Here's the drawing with two shaded views (mm, measured from the low corner). I have some questions. A direction names the side the tool comes from. Round coordinates to 2 decimals unless told otherwise and drop trailing zeros. Loops run counter-clockwise (first coordinate to the right, second up) from the corner with the lowest first, then second, coordinate; pieces in that order, holes last.
(1) Thinking about a two-plate mould opening in Z: for the marked faces 3, 4, 5 and 6, which applies, released by +Z, released by -Z, zero draft, split by the parting line, or undercut?
(2) I want a section at A-A on z = 12.7. Write out the boundary of the cut face in (x, y) (3 decimals).
(3) I want a section at B-B on y = 38. Write out the boundary of the cut face in (x, z) (3 decimals).
(4) If I drill on line 1 along Y through (x, z) = (24.25, 12); line 2 along X through (y, z) = (46.5, 7) (3 decimals); line 3 along Y through (x, z) = (26.5, 11), over which ranges is the centre line in solid material (lowest first)?
(5) I want a section at C-C on x = 12. Write out the boundary of the cut face in (y, z).
(6) Will these pins go through, and if not, where does the flat tip stop? pin 1 Ø7.5 at (y, z) = (48.5, 11.5) entering from -X; pin 2 Ø4 at (x, z) = (24, 12) entering from -Y; pin 3 Ø7.5 at (x, z) = (6.5, 12.5) entering from +Y.
(7) I want a section at D-D on z = 23.25. Write out the boundary of the cut face in (x, y) (3 decimals).
(8) Which directions (+Z, -Z, +X, -X, +Y, -Y) give clear straight access to the entire face, cutting with the end or side of a thin tool? Please do the marked faces 1 and 2.
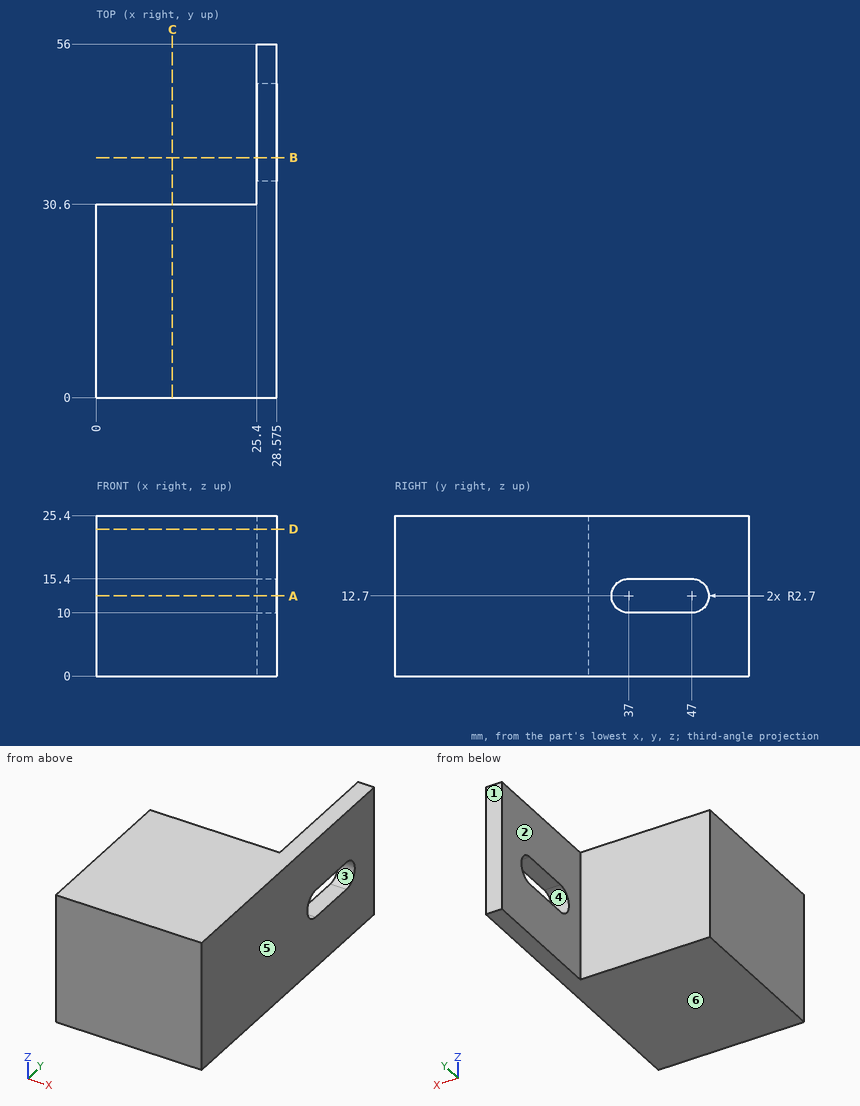
Filled sheet:
1. face 3: undercut
1. face 4: undercut
1. face 5: zero draft
1. face 6: released by -Z
2. outline: (0, 0) - (28.575, 0) - (28.575, 34.3) - (25.4, 34.3) - (25.4, 30.6) - (0, 30.6) - close; (25.4, 49.7) - (28.575, 49.7) - (28.575, 56) - (25.4, 56) - close
3. outline: (25.4, 0) - (28.575, 0) - (28.575, 10) - (25.4, 10) - close; (25.4, 15.4) - (28.575, 15.4) - (28.575, 25.4) - (25.4, 25.4) - close
4. line 1: y = 0 to 30.6
4. line 2: x = 25.4 to 28.575
4. line 3: y = 0 to 34.9, 49.1 to 56
5. outline: (0, 0) - (30.6, 0) - (30.6, 25.4) - (0, 25.4) - close
6. pin 1: stops at x = 25.4
6. pin 2: stops at y = 0
6. pin 3: stops at y = 30.6
7. outline: (0, 0) - (28.575, 0) - (28.575, 56) - (25.4, 56) - (25.4, 30.6) - (0, 30.6) - close
8. face 1: +Z, -Z, +X, -X, +Y
8. face 2: +Z, -Z, -X, +Y
